Could you check a few things on this drawing? It's one solid part, dimensions in mm from its lowest x, y, z. A direction names the side the tool comes from. Give positions to 0.01 mm unless a question says otherwise; leave off trailing zeros. Loops run counter-clockwise (first coordinate to the right, second up) from the corner with the lowest first, then second, coordinate; pieces in that order, holes last. Notation, with made-up numbers: (8, 24) - (38, 24) arc R23 ccw to (38, 54) - close; hole circle Ø1 at (54, -20.75). An arc over 180 degrees is marked (long way). Put each result on its own line as item: value. Start each with the question number.
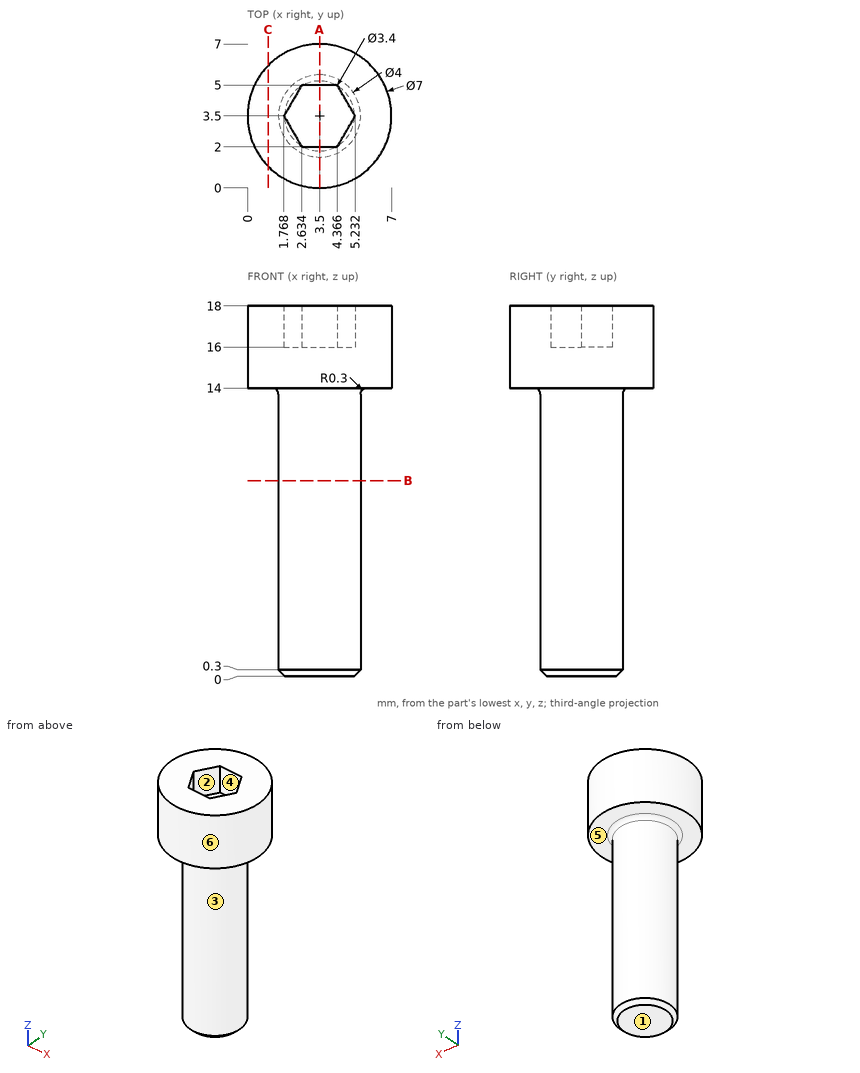
1) Suppose I cut it at A-A on x = 3.5. Please give me the cut outline in (y, z).
2) Suppose I cut it at B-B on z = 9.5. Please give me the cut outline in (x, y).
3) Which directions (+Z, -Z, +X, -X, +Y, -Y) give clear straight access to the entire face, cutting with the end or side of a thin tool? Please do the marked faces 4, 5 and 6.
4) I need wall thicknesses on line 1 (Z direction, x = 3, y = 6.5); line 2 (Y direction, x = 4.5, z = 13); line 3 (Z direction, x = 3.75, y = 2.5). Which ranges of each line are inside material? Lowest first, please.
5) Thinking about a two-plate mould opening in Y: for the marked faces 1, 2 and 3, which applies, pulls with the +Y half, pulls with the -Y half, needs draft (parallel to the pull), parting line crosses it, or undercut?
6) I'm going to push flat-ended pins straight in: P1, Ø1.5, axis at x = 2.5, z = 3.5, coming from the -Y side; P2, Ø1.5, axis at y = 6, z = 2.5, coming from the -X side; P3, Ø4, axis at y = 5.5, z = 3, coming from the -X side. Where does each tip first touch, or does it pass through?
7) Suppose I cut it at C-C on x = 1. Please give me the cut outline in (y, z), plus the area to 3 significant figures.
Ans:
1. outline: (0, 14) - (1.2, 14) arc R0.3 cw to (1.5, 13.7) - (1.5, 0.3) - (1.8, 0) - (5.2, 0) - (5.5, 0.3) - (5.5, 13.7) arc R0.3 cw to (5.8, 14) - (7, 14) - (7, 18) - (5, 18) - (5, 16) - (2, 16) - (2, 18) - (0, 18) - close
2. outline: circle Ø4 at (3.5, 3.5)
3. face 4: +Z
3. face 5: -Z
3. face 6: +Z, -Z
4. line 1: z = 14 to 18
4. line 2: y = 1.77 to 5.23
4. line 3: z = 0 to 16
5. face 1: needs draft
5. face 2: undercut
5. face 3: parting line crosses it
6. P1: stops at y = 1.52
6. P2: stops at x = 2.53
6. P3: stops at x = 1.5
7. outline: (1.05, 14) - (5.95, 14) - (5.95, 18) - (1.05, 18) - close
7. area: 19.6 mm²
